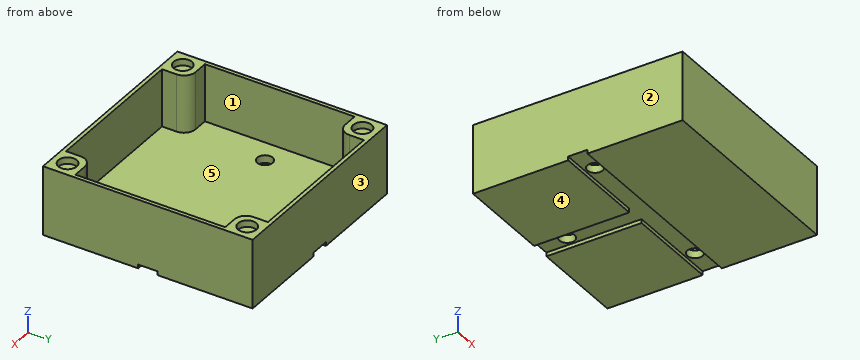
```python
from build123d import *

# Parameters (mm, degrees)
SKICA1_W                 = 54.6
SKICA1_H                 = 54.6
P_IDAT_VYSUNUT_M2_DEPTH  = 3
SKICA5_W                 = 5
SKICA5_H                 = 24.8
SKICA5_W_2               = 54.6
SKICA5_H_2               = 5
ODEBRAT_VYSUNUT_M3_DEPTH = 1
SKICA14_W                = 52.6
SKICA14_H                = 1
P_IDAT_VYSUNUT_M9_DEPTH  = 15
SKICA17_R                = 2
ODEBRAT_VYSUNUT_M8_DEPTH = 7
SKICA19_W                = 7.8
SKICA19_H                = 7.8
P_IDAT_VYSUNUT_M10_DEPTH = 18
SKICA20_R                = 2.4
ODEBRAT_VYSUNUT_M9_DEPTH = 1.7
ZAOBLIT1_R               = 3


with BuildPart() as part:
    # Skica1 → Přidat vysunutím2 (new body)
    with BuildSketch(Plane.XY):
        Rectangle(SKICA1_W, SKICA1_H)
    extrude(amount=P_IDAT_VYSUNUT_M2_DEPTH)

    # Skica5 → Odebrat vysunutím3 (cut)
    with BuildSketch(Plane(origin=(0, 0, 0), x_dir=(-1, 0, 0), z_dir=(0, 0, -1))):
        with Locations((0, 14.9)):
            Rectangle(SKICA5_W, SKICA5_H)
        Rectangle(SKICA5_W_2, SKICA5_H_2)
    extrude(amount=-ODEBRAT_VYSUNUT_M3_DEPTH, mode=Mode.SUBTRACT)

    # Skica14 → Přidat vysunutím9 (add)
    with BuildSketch(Plane.XY.offset(3)):
        Polygon((27.3, 27.3), (-27.3, 27.3), (-27.3, -27.3), (-26.3, -27.3), (-26.3, -26.3), (-26.3, 26.3), (26.3, 26.3), (26.3, -26.3), (26.3, -27.3), (27.3, -27.3), align=None)
        with Locations((0, -26.8)):
            Rectangle(SKICA14_W, SKICA14_H)
    extrude(amount=P_IDAT_VYSUNUT_M9_DEPTH)

    # Skica17 → Odebrat vysunutím8 (cut)
    with BuildSketch(Plane(origin=(0, 0, 1), x_dir=(-1, 0, 0), z_dir=(0, 0, -1))):
        with Locations((-20.3, 0)):
            Circle(SKICA17_R)
        with Locations((20.3, 0)):
            Circle(SKICA17_R)
        with Locations((0, 20.3)):
            Circle(SKICA17_R)
    extrude(amount=-ODEBRAT_VYSUNUT_M8_DEPTH, mode=Mode.SUBTRACT)

    # Skica19 → Přidat vysunutím10 (add)
    with BuildSketch(Plane(origin=(0, 0, 0), x_dir=(-1, 0, 0), z_dir=(0, 0, -1))):
        with Locations((-23.4, 23.4)):
            Rectangle(SKICA19_W, SKICA19_H)
        with Locations((23.4, 23.4)):
            Rectangle(SKICA19_W, SKICA19_H)
        with Locations((-23.4, -23.4)):
            Rectangle(SKICA19_W, SKICA19_H)
        with Locations((23.4, -23.4)):
            Rectangle(SKICA19_W, SKICA19_H)
    extrude(amount=-P_IDAT_VYSUNUT_M10_DEPTH)

    # Skica20 → Odebrat vysunutím9 (cut)
    with BuildSketch(Plane.XY.offset(18)):
        with Locations((-23.4, -23.4)):
            Circle(SKICA20_R)
        with Locations((-23.4, 23.4)):
            Circle(SKICA20_R)
        with Locations((23.400280565, 23.4)):
            Circle(SKICA20_R)
        with Locations((23.400280565, -23.4)):
            Circle(SKICA20_R)
    extrude(amount=-ODEBRAT_VYSUNUT_M9_DEPTH, mode=Mode.SUBTRACT)

    # Zaoblit1
    zaoblit1_edges = [part.edges().sort_by_distance(p)[0] for p in [
        (-19.5, 19.5, 10.5),
        (19.5, -19.5, 10.5),
        (-19.5, -19.5, 10.5),
        (19.5, 19.5, 10.5),
    ]]
    fillet(zaoblit1_edges, radius=ZAOBLIT1_R)


solid = part.part
```
Here's how the part is built. I have some questions about the finished solid (model axes, mm). Face numbers are marked on the shaded views. A direction names the side the tool comes from. Round coordinates to 2 decimals unless told otherwise and drop trailing zeros. Order: outer loops, then holes, each group sorted by start corner. A loop starts at its lowest first (then second) coordinate and runs counter-clockwise, first axis right, second up. Notation, with made-up numbers: (85, 39) -> (117, 39) arc R12 ccw to (117, 49) -> close; hole circle Ø7 at (20, -5). An arc over 180 degrees is marked (long way). Use a Markdown table: item, result. Add a question column.
(1) Suppose I cut it at A-A, the plane y = 0. Please give me the cut outline in (x, z).
(2) For pin 1 Ø15 at (x, y) = (-13.5, 11.5) entering from -Z; pin 2 Ø1.4 at (x, y) = (-24, 23.5) entering from +Z; pin 3 Ø1.5 at (x, y) = (13.5, -3.5) entering from +Z; pin 4 Ø3 at (x, y) = (-20.3, 0) entering from +Z, each with a flat end and sliding along its axis, tell me the tip position at first contact or that it passes through.
(3) I need wall thicknesses on line 1 along Y through (x, z) = (15.5, 5.5); line 2 along Y through (x, z) = (20.3, 1.95). Which ranges of each line are inside material? Lowest first, please.
(4) Suppose I cut it at B-B, the plane x = 0. Please give me the cut outline in (y, z), and give its area (3 significant figures).
(5) Suppose I cut it at C-C, the plane z = 15.5. Please give me the cut outline in (x, y), and give its area (3 significant figures).
(6) If we mould it in two halves opening along Y, with no side actions, what happens to the marked faces 3, 4 and 5? For each: released by +Y, released by -Y, zero draft, split by the parting line, or undercut.
(7) Suppose I cut it at D-D, the plane x = 8. Please give me the cut outline in (y, z), and give its area (3 significant figures).
(8) For the marked faces 1 and 2, which set-ups out of +Z, -Z, +X, -X, +Y, -Y let a thin tool reach every point of the face, with its end or its side?
Verdict:
| question | item | result |
|---|---|---|
| 1 | outline | (-27.3, 1) -> (-22.3, 1) -> (-22.3, 3) -> (-26.3, 3) -> (-26.3, 18) -> (-27.3, 18) -> close; (-18.3, 1) -> (18.3, 1) -> (18.3, 3) -> (-18.3, 3) -> close; (22.3, 1) -> (27.3, 1) -> (27.3, 18) -> (26.3, 18) -> (26.3, 3) -> (22.3, 3) -> close |
| 2 | pin 1 | z = 0 |
| 2 | pin 2 | z = 16.3 |
| 2 | pin 3 | z = 3 |
| 2 | pin 4 | through |
| 3 | line 1 | -27.3 to -26.3, 26.3 to 27.3 |
| 3 | line 2 | -27.3 to -2, 2 to 27.3 |
| 4 | outline | (-27.3, 0) -> (-2.5, 0) -> (-2.5, 1) -> (18.3, 1) -> (18.3, 3) -> (-26.3, 3) -> (-26.3, 18) -> (-27.3, 18) -> close; (22.3, 1) -> (27.3, 1) -> (27.3, 18) -> (26.3, 18) -> (26.3, 3) -> (22.3, 3) -> close |
| 4 | area | 156 mm2 |
| 5 | outline | (-27.3, -27.3) -> (27.3, -27.3) -> (27.3, 27.3) -> (-27.3, 27.3) -> close; hole (-26.3, -19.5) -> (-22.5, -19.5) arc R3 cw to (-19.5, -22.5) -> (-19.5, -26.3) -> (19.5, -26.3) -> (19.5, -22.5) arc R3 cw to (22.5, -19.5) -> (26.3, -19.5) -> (26.3, 19.5) -> (22.5, 19.5) arc R3 cw to (19.5, 22.5) -> (19.5, 26.3) -> (-19.5, 26.3) -> (-19.5, 22.5) arc R3 cw to (-22.5, 19.5) -> (-26.3, 19.5) -> close |
| 5 | area | 392 mm2 |
| 6 | face 3 | released by +Y |
| 6 | face 4 | zero draft |
| 6 | face 5 | undercut |
| 7 | outline | (-27.3, 0) -> (-2.5, 0) -> (-2.5, 1) -> (2.5, 1) -> (2.5, 0) -> (27.3, 0) -> (27.3, 18) -> (26.3, 18) -> (26.3, 3) -> (-26.3, 3) -> (-26.3, 18) -> (-27.3, 18) -> close |
| 7 | area | 189 mm2 |
| 8 | face 1 | +Z |
| 8 | face 2 | +Z, -Z, -X, +Y, -Y |
